from build123d import *

# Parameters (mm, degrees)
F0_R     = 6.05
F1_DEPTH = 39
F3_D     = 6


with BuildPart() as f1:
    # F0 (on Right) → F1 (new body)
    with BuildSketch(Plane.YZ):
        with BuildLine():
            Line((6.614378, 7.5), (-6.614378, 7.5))
            ThreePointArc((-6.614378, 7.5), (0, -10), (6.614378, 7.5))
        make_face()
        Circle(F0_R, mode=Mode.SUBTRACT)
    extrude(amount=F1_DEPTH)

    # F3 (through all)
    with Locations(Plane.XY.offset(7.5)):
        with Locations((6, 0), (33, 0)):
            Hole(F3_D / 2)


solid = f1.part
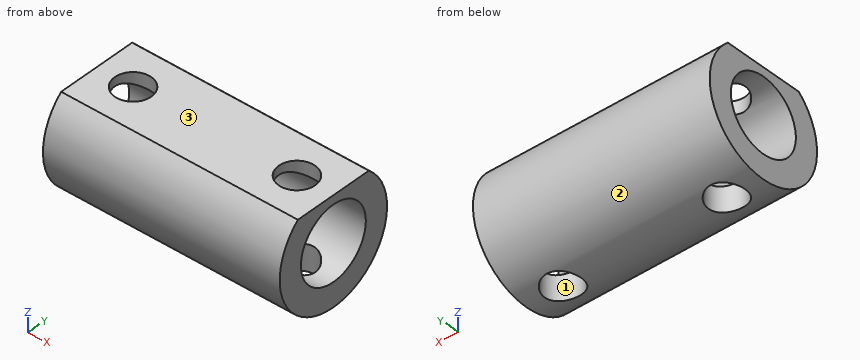
The model under review builds one solid part; all positions refer to its coordinate system, in mm. Face numbers are marked on the shaded views. Coordinates: 2 decimals unless noted, no trailing zeros. Loops run counter-clockwise (first coordinate to the right, second up) from the corner with the lowest first, then second, coordinate; pieces in that order, holes last. Notation, with made-up numbers: (-37.75, 15) -> (-12.75, 15) arc R26 ccw to (-12.75, 39) -> close; hole circle Ø6 at (45.25, 8.5). An arc over 180 degrees is marked (long way). Use a Markdown table: item, result. Add a question column.
1. Add section B-B on z = 3. Write out the cut boundary in (x, y).
2. Clearance check with flat-ended pins moving along their axes: pin 1 Ø2 at (x, y) = (4.5, -7) entering from -Z; pin 2 Ø4 at (x, z) = (32.5, -3.5) entering from -Y; pin 3 Ø1 at (x, z) = (34, -2.5) entering from +Y. State where each tip first meets the part, or that it passes through.
3. Draft analysis for pull direction Y (two halves, no side actions). For the marked faces 1, 2 and 3, state which applies: pulls with the +Y half, pulls with the -Y half, needs draft (parallel to the pull), parting line crosses it, or undercut.
4. Add section A-A on y = 0. Write out the cut boundary in (x, z), plus the area to 3 significant figures.
5. Add section C-C on x = 7.5. Write out the cut boundary in (y, z), plus the area to 3 significant figures.
6. Add section D-D on y = -5.25. Write out the cut boundary in (x, z).
7. To check wall thickness, follow line 1 (X direction, y = 0, z = -7.3); line 2 (Z direction, x = 26.5, y = 0); line 3 (Y direction, x = 6, z = 5.9). State the ranges of each line that lie inside material, in increasing order.
Returned:
| question | item | result |
|---|---|---|
| 1 | outline | (0, -9.54) -> (39, -9.54) -> (39, -5.25) -> (0, -5.25) -> close; (0, 5.25) -> (39, 5.25) -> (39, 9.54) -> (0, 9.54) -> close |
| 2 | pin 1 | stops at z = -8 |
| 2 | pin 2 | stops at y = -9.89 |
| 2 | pin 3 | stops at y = 9.8 |
| 3 | face 1 | undercut |
| 3 | face 2 | parting line crosses it |
| 3 | face 3 | needs draft |
| 4 | outline | (0, -10) -> (3, -10) -> (3, -6.05) -> (0, -6.05) -> close; (0, 6.05) -> (3, 6.05) -> (3, 7.5) -> (0, 7.5) -> close; (9, -10) -> (30, -10) -> (30, -6.05) -> (9, -6.05) -> close; (9, 6.05) -> (30, 6.05) -> (30, 7.5) -> (9, 7.5) -> close; (36, -10) -> (39, -10) -> (39, -6.05) -> (36, -6.05) -> close; (36, 6.05) -> (39, 6.05) -> (39, 7.5) -> (36, 7.5) -> close |
| 4 | area | 146 mm² |
| 5 | outline | (-6.61, 7.5) arc R10 ccw to (-2.6, -9.66) -> (-2.6, -5.46) arc R6.05 cw to (-2.6, 5.46) -> (-2.6, 7.5) -> close; (2.6, -9.66) arc R10 ccw to (6.61, 7.5) -> (2.6, 7.5) -> (2.6, 5.46) arc R6.05 cw to (2.6, -5.46) -> close |
| 5 | area | 147 mm² |
| 6 | outline | (0, -8.51) -> (39, -8.51) -> (39, -3.01) -> (0, -3.01) -> close; (0, 3.01) -> (39, 3.01) -> (39, 7.5) -> (0, 7.5) -> close |
| 7 | line 1 | x = 0 to 3, 9 to 30, 36 to 39 |
| 7 | line 2 | z = -10 to -6.05, 6.05 to 7.5 |
| 7 | line 3 | y = -8.07 to -3, 3 to 8.07 |
